Print and shaded views of the part. All mm, measured from the part's lowest x, y and z. A direction names the side the tool comes from. Give positions to 0.01 mm unless a question says otherwise; leave off trailing zeros. Loops run counter-clockwise (first coordinate to the right, second up) from the corner with the lowest first, then second, coordinate; pieces in that order, holes last.
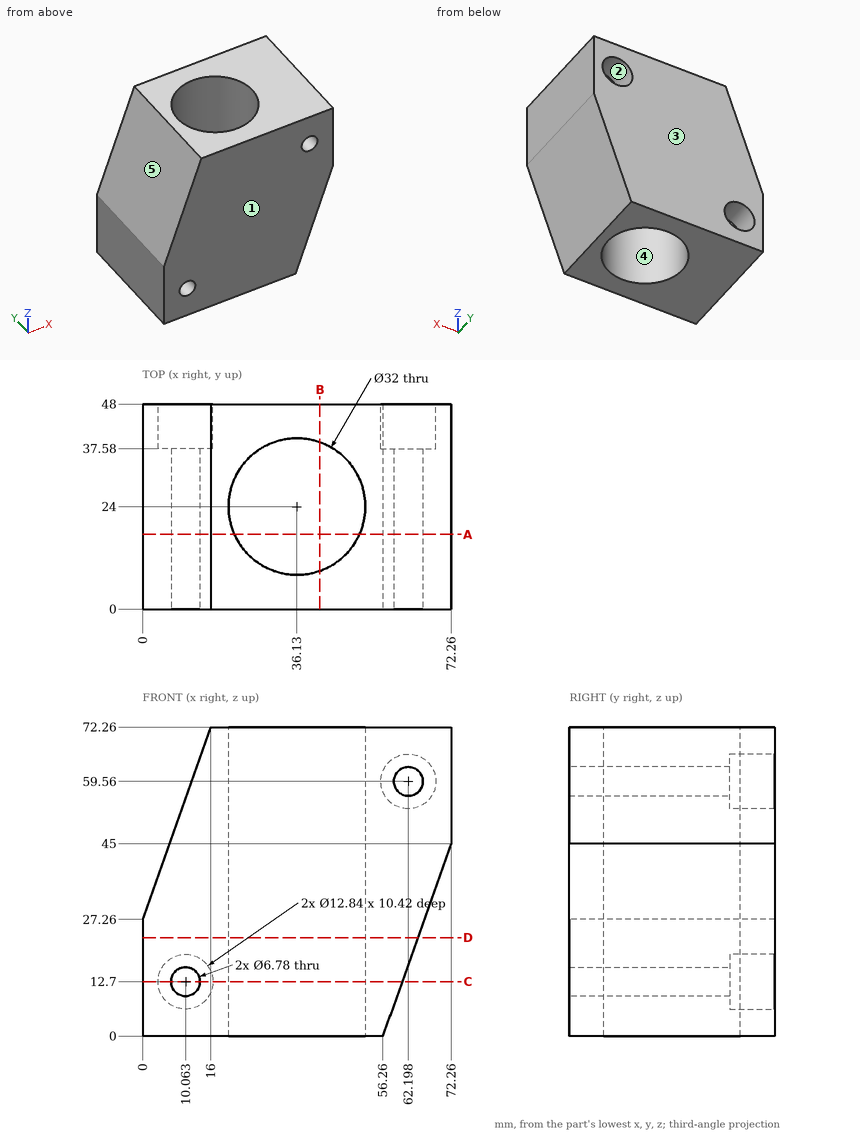
1. Saw through at D-D, the plane z = 23. List the corners of the cut face in (x, y), and give its area (3 significant figures).
Responses:
outline: (0, 0) - (64.44, 0) - (64.44, 48) - (0, 48) - close; hole circle Ø32 at (36.13, 24)
area: 2,290 mm2
2. Saw through at A-A, the plane y = 17.5. List the corners of the cut face in (x, z), and give its area (3 significant figures).
Responses:
outline: (0, 0) - (21.51, 0) - (21.51, 72.26) - (16, 72.26) - (0, 27.26) - close; (50.75, 0) - (56.26, 0) - (72.26, 45) - (72.26, 72.26) - (50.75, 72.26) - close; hole circle Ø6.78 at (10.06, 12.7); hole circle Ø6.78 at (62.2, 59.56)
area: 2,320 mm2
3. Tool access for the marked faces 1 and 2: list every direction of +Z, -Z, +X, -X, +Y, -Y with a clear straight run to the whole face (end or side of a thin tool).
Responses:
face 1: +Z, -Z, +X, -X, -Y
face 2: +Y
4. Pull direction X, two halves, no side cores. Call the marked faces 3, 4 and 5: released by +X, released by -X, zero draft, split by the parting line, or undercut.
Responses:
face 3: zero draft
face 4: undercut
face 5: released by -X
5. Saw through at B-B, the plane x = 41.5. List the corners of the cut face in (y, z).
Responses:
outline: (0, 0) - (8.93, 0) - (8.93, 72.26) - (0, 72.26) - close; (39.07, 0) - (48, 0) - (48, 72.26) - (39.07, 72.26) - close
6. Probe line 1 along Y through (x, z) = (36.13, 33); line 2 along X through (y, z) = (27.5, 59.56) (1 decimal); line 3 along X through (y, z) = (22.5, 12.7) (1 decimal). List the from-to ranges inside material, lowest first.
Responses:
line 1: y = 0 to 8, 40 to 48
line 2: x = 11.5 to 20.5, 51.7 to 58.8, 65.6 to 72.3
line 3: x = 0 to 6.7, 13.5 to 20.2, 52.1 to 60.8
7. Drop a flat-ended pin along its axis: pin 1 (10.5 mm diameter, centred on x = 10.06, z = 12.7, fed in from +Y). Give the stop position or say it passes through.
Responses:
pin 1: stops at y = 37.58
8. Saw through at C-C, the plane z = 12.7. List the corners of the cut face in (x, y) (1 decimal).
Responses:
outline: (0, 0) - (6.7, 0) - (6.7, 37.6) - (3.6, 37.6) - (3.6, 48) - (0, 48) - close; (13.5, 0) - (60.8, 0) - (60.8, 48) - (16.5, 48) - (16.5, 37.6) - (13.5, 37.6) - close; hole circle Ø32 at (36.1, 24)
